Build history of the part. All positions in model axes, mm. Round coordinates to 2 decimals unless told otherwise and drop trailing zeros. Write each loop counter-clockwise with the first axis right and the second up, starting at its lowest first coordinate (ties: lowest second). Pieces come first, ordered by that corner, then holes.
Item 1: Band-saw the part on C-C, the plane y = 31.5. Write the cut outline in (x, z), then the cut area to 3 significant figures.
Item 2: Wall check: probe 1 along X at (y, z) = (27, 0); probe 2 along X at (y, z) = (3.5, -1); probe 3 along Z at (x, y) = (9.5, 32). Give the ranges that are in metal, low to high.
Item 3: Band-saw the part on B-B, the plane z = 0. Write the cut outline in (x, y), then the cut area to 3 significant figures.
Item 4: Band-saw the part on A-A, the plane x = 0. Write the cut outline in (y, z), then the cut area to 3 significant figures.
Item 5: Drop flat-ended pins along their axis: pin 1 Ø3 at (x, y) = (-16, 15) entering from +Z; pin 2 Ø2 at (y, z) = (6.5, -16.5) entering from +X; pin 3 Ø10 at (x, y) = (16, 20.5) entering from +Z. Give the stop position or say it passes through.
```python
from build123d import *

# Parameters (mm, degrees)
SKETCH1_R           = 22.5
BOSS_EXTRUDE1_DEPTH = 40.278278
SKETCH2_R           = 14.06292986
CUT_EXTRUDE1_DEPTH  = 52.330689443
CHAMFER1_SIZE       = 2.746557


with BuildPart() as part:
    # Sketch1 → Boss-Extrude1 (new body)
    with BuildSketch(Plane(origin=(0, 0, 0), x_dir=(1, 0, 0), z_dir=(0, 1, 0))):
        with Locations(Location((0, 0, 0), (0, 0, 270))):
            Circle(SKETCH1_R)
    extrude(amount=BOSS_EXTRUDE1_DEPTH)

    # Sketch2 → Cut-Extrude1 (cut, through all)
    with BuildSketch(Plane(origin=(0, 0, 0), x_dir=(1, 0, 0), z_dir=(0, 1, 0))):
        with Locations(Location((0, 0, 0), (0, 0, 270))):
            Circle(SKETCH2_R)
    extrude(amount=CUT_EXTRUDE1_DEPTH, mode=Mode.SUBTRACT)

    # Chamfer1
    chamfer1_edges = [part.edges().sort_by_distance(p)[0] for p in [
        (0, 0, -22.5),
        (0, 40.278278, -22.5),
        (0, 0, -14.06292986),
        (0, 40.278278, -14.06292986),
    ]]
    chamfer(chamfer1_edges, length=CHAMFER1_SIZE)


solid = part.part
```
Results:
1. outline: circle Ø45 at (0, 0); hole circle Ø28.13 at (0, 0)
1. area: 969 mm2
2. probe 1: x = -22.5 to -14.06, 14.06 to 22.5
2. probe 2: x = -22.48 to -14.03, 14.03 to 22.48
2. probe 3: z = -20.4 to -10.37, 10.37 to 20.4
3. outline: (-22.5, 2.75) - (-19.75, 0) - (-16.81, 0) - (-14.06, 2.75) - (-14.06, 37.53) - (-16.81, 40.28) - (-19.75, 40.28) - (-22.5, 37.53) - close; (14.06, 2.75) - (16.81, 0) - (19.75, 0) - (22.5, 2.75) - (22.5, 37.53) - (19.75, 40.28) - (16.81, 40.28) - (14.06, 37.53) - close
3. area: 649 mm2
4. outline: (0, -19.75) - (2.75, -22.5) - (37.53, -22.5) - (40.28, -19.75) - (40.28, -16.81) - (37.53, -14.06) - (2.75, -14.06) - (0, -16.81) - close; (0, 16.81) - (2.75, 14.06) - (37.53, 14.06) - (40.28, 16.81) - (40.28, 19.75) - (37.53, 22.5) - (2.75, 22.5) - (0, 19.75) - close
4. area: 649 mm2
5. pin 1: stops at z = 17.2
5. pin 2: stops at x = 16.31
5. pin 3: stops at z = 19.63
